Model file for the job. Use its own axes, mm. Face numbers are marked on the shaded views. A direction names the side the tool comes from. Round coordinates to 2 decimals unless told otherwise and drop trailing zeros. Write each loop counter-clockwise with the first axis right and the second up, starting at its lowest first coordinate (ties: lowest second). Pieces come first, ordered by that corner, then holes. Notation, with made-up numbers: (33, 26.5) - (90, 26.5) arc R23 cw to (90, 47.5) - close; hole circle Ø10 at (-16.5, -1.5). An arc over 180 degrees is marked (long way). Answer as a JSON object with one key per item and string values. Group by question number.
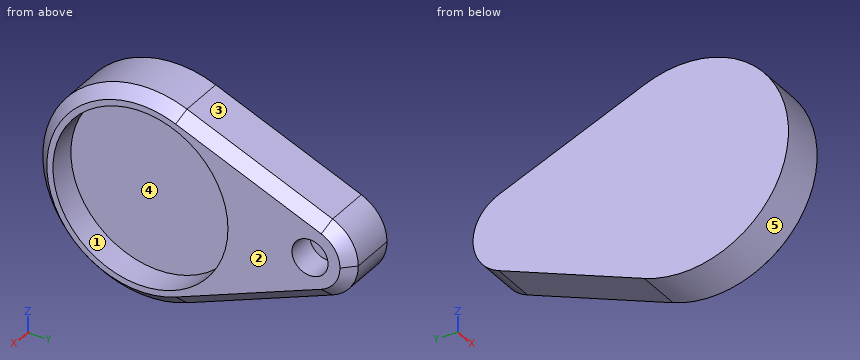
from build123d import *

# Parameters (mm, degrees)
F1_DEPTH = 25.4
F2_R     = 39.820498
F3_DEPTH = 12.7
F4_R     = 8.210642
F5_DEPTH = 12.7
F6_SIZE  = 5.08


with BuildPart() as f1:
    # F0 (on Right) → F1 (new body)
    with BuildSketch(Plane.YZ):
        with BuildLine():
            ThreePointArc((17.909064, -44.198928), (39.549668, -26.647768), (47.68941, 0))
            ThreePointArc((47.68941, 0), (39.549668, 26.647768), (17.909064, 44.198928))
            ThreePointArc((17.909064, 44.198928), (-47.68941, 0), (17.909064, -44.198928))
        make_face()
        with BuildLine():
            ThreePointArc((17.909064, 44.198928), (39.549668, 26.647768), (47.68941, 0))
            ThreePointArc((47.68941, 0), (39.549668, -26.647768), (17.909064, -44.198928))
            Line((17.909064, -44.198928), (84.17689, -17.347717))
            ThreePointArc((84.17689, -17.347717), (58.430027, 0), (84.17689, 17.347717))
            Line((84.17689, 17.347717), (17.909064, 44.198928))
        make_face()
        with BuildLine():
            ThreePointArc((95.865432, 0), (92.67065, 10.459031), (84.17689, 17.347717))
            ThreePointArc((84.17689, 17.347717), (58.430027, 0), (84.17689, -17.347717))
            ThreePointArc((84.17689, -17.347717), (92.67065, -10.459031), (95.865432, 0))
        make_face()
    extrude(amount=F1_DEPTH)

    # F2 (on face) → F3 (cut)
    with BuildSketch(Plane.YZ.offset(25.4)):
        Circle(F2_R)
    extrude(amount=-F3_DEPTH, mode=Mode.SUBTRACT)

    # F4 (on face) → F5 (cut)
    with BuildSketch(Plane.YZ.offset(25.4)):
        with Locations((77.147729, 0)):
            Circle(F4_R)
    extrude(amount=-F5_DEPTH, mode=Mode.SUBTRACT)

    # F6
    f6_edges = [f1.edges().sort_by_distance(p)[0] for p in [
        (25.4, 51.042977, 30.773322),
    ]]
    chamfer(f6_edges, length=F6_SIZE)


solid = f1.part
(1) Slice it at B-B (y = 0). Write the cut outline in (x, z), then the cut area to 3 significant figures.
(2) Slice it at C-C (x = 4). Write the cut outline in (y, z), then the cut area to 3 significant figures.
(3) Drill centre lines: line 1 (Y direction, x = 14, z = -6); line 2 (Z direction, x = 13.75, y = 0.5); line 3 (Y direction, x = 23.25, z = -1.5). Where is each one in solid material? Low to high. Write a range as from..to.
(4) Flat gauge pins, fed straight in: pin 1 (10 mm diameter, centred on x = 20, z = 24, fed in from +Y); pin 2 (12 mm diameter, centred on x = 7.5, z = -1.5, fed in from -Y); pin 3 (12 mm diameter, centred on x = 13.5, y = 34, fed in from -Z). Where does each tip first touch, or does it go through?
(5) Slice it at A-A (x = 15.75). Write the cut outline in (y, z), then the cut area to 3 significant figures.
(6) 3-axis set-ups, long thin cutter, end or side, ignore diameter. For the marked faces 4 and 5: which of +Z, -Z, +X, -X, +Y, -Y reach the whole face in a straight line?
(7) Pull direction Y, two halves, no side cores. Call the marked faces 1, 2 and 3: pulls with the +Y half, pulls with the -Y half, needs draft (parallel to the pull), parting line crosses it, or undercut.
(8) Slice it at D-D (y = 58). Write the cut outline in (x, z), then the cut area to 3 significant figures.
Answer:
{
 "1": {"outline": "(0, -47.69) - (20.32, -47.69) - (25.4, -42.61) - (25.4, -39.82) - (12.7, -39.82) - (12.7, 39.82) - (25.4, 39.82) - (25.4, 42.61) - (20.32, 47.69) - (0, 47.69) - close", "area": "1,390 mm²"},
 "2": {"outline": "(17.91, -44.2) - (84.18, -17.35) arc R18.72 ccw to (84.18, 17.35) - (17.91, 44.2) arc R47.69 ccw (long way) to start", "area": "9,610 mm²"},
 "3": {"line 1": "-47.31..-39.37, 39.37..71.54, 82.75..94.88", "line 2": "-47.69..-39.82, 39.82..47.69", "line 3": "-44.73..-39.79, 39.79..69.08, 85.22..92.86"},
 "4": {"pin 1": "y = 80.1", "pin 2": "y = -47.69", "pin 3": "z = -40.11"},
 "5": {"outline": "(17.91, -44.2) - (84.18, -17.35) arc R18.72 ccw to (84.18, 17.35) - (17.91, 44.2) arc R47.69 ccw (long way) to start; hole circle Ø79.64 at (0, 0); hole circle Ø16.42 at (77.15, 0)", "area": "4,420 mm²"},
 "6": {"face 4": "+X", "face 5": "+X, -X"},
 "7": {"face 1": "undercut", "face 2": "needs draft", "face 3": "pulls with the +Y half"},
 "8": {"outline": "(0, -27.95) - (20.32, -27.95) - (25.4, -22.47) - (25.4, 22.47) - (20.32, 27.95) - (0, 27.95) - close", "area": "1,390 mm²"}
}
